Job drawing, mm, ordinate dimensions from the low corner. One solid piece. A direction names the side the tool comes from. Round coordinates to 2 decimals unless told otherwise and drop trailing zeros. Write each loop counter-clockwise with the first axis right and the second up, starting at its lowest first coordinate (ties: lowest second). Pieces come first, ordered by that corner, then holes.
1) Saw through at A-A (y = 50). Write the cut outline in (x, z) (1 decimal).
2) Wall check: probe 1 along Y at (x, z) = (6, 28.5); probe 2 along Z at (x, y) = (29, 59) (1 decimal); probe 3 along Z at (x, y) = (14.5, 32) (1 decimal). Give the ranges that are in metal, low to high.
3) Pull direction X, two halves, no side cores. Call the marked faces 5, 6 and 7: +X half, -X half, draft (parallel to the pull), parting line (faces both ways), or undercut.
4) Which spindle directions (+Z, -Z, +X, -X, +Y, -Y) get a long thin tool onto all of the face, cutting with end or side? Do the marked faces 1, 2, 3 and 4. Say none if no direction does.
5) Saw through at D-D (x = 5). Write the cut outline in (y, z) (1 decimal).
6) Saw through at C-C (z = 31). Write the cut outline in (x, y) (1 decimal), plus the area to 3 significant figures.
7) Flat gauge pins, fed straight in: pin 1 (3 mm diameter, centred on y = 16.5, z = 20, fed in from +X) (1 decimal); pin 2 (9 mm diameter, centred on x = 20, y = 25, fed in from +Z); pin 3 (6 mm diameter, centred on x = 5, y = 56, fed in from -Z). Where does each tip first touch, or does it go through?
8) Saw through at B-B (x = 17.5). State how many separate pieces and enclosed holes the cut face has.
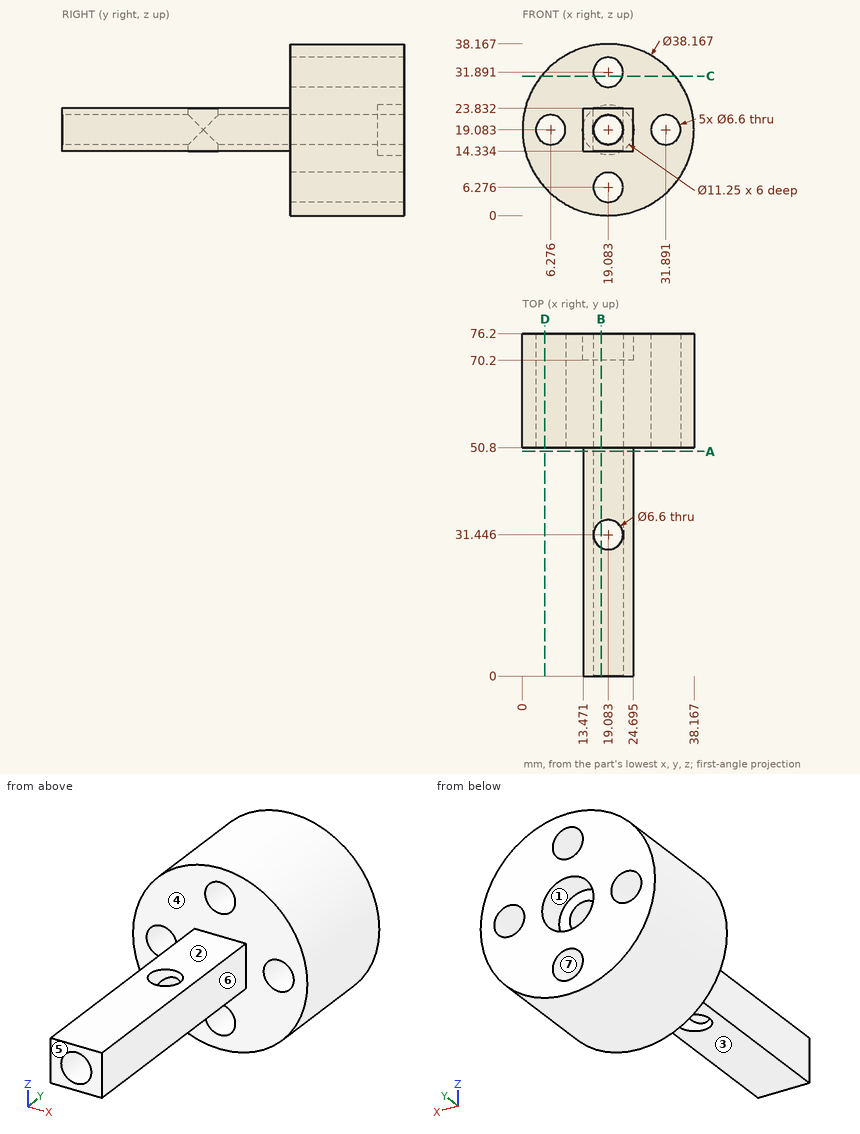
Evaluation:
1. outline: (13.5, 14.3) - (24.7, 14.3) - (24.7, 23.8) - (13.5, 23.8) - close; hole circle Ø6.6 at (19.1, 19.1)
2. probe 1: y = 50.8 to 76.2
2. probe 2: z = 2.8 to 17.5, 20.7 to 35.4
2. probe 3: z = 14.3 to 23.8
3. face 5: draft
3. face 6: +X half
3. face 7: undercut
4. face 1: +Y
4. face 2: +Z, +X, -X, -Y
4. face 3: -Z, +X, -X, -Y
4. face 4: -Y
5. outline: (50.8, 6.2) - (76.2, 6.2) - (76.2, 16) - (50.8, 16) - close; (50.8, 22.1) - (76.2, 22.1) - (76.2, 32) - (50.8, 32) - close
6. outline: (4.2, 50.8) - (15.9, 50.8) - (15.9, 76.2) - (4.2, 76.2) - close; (22.3, 50.8) - (34, 50.8) - (34, 76.2) - (22.3, 76.2) - close
6. area: 596 mm2
7. pin 1: stops at x = 24.7
7. pin 2: stops at z = 23.83
7. pin 3: stops at z = 3.55
8. separate pieces: 6
8. enclosed holes: 0
